Read the model definition and answer for the solid it produces. Units are mm, in the model's axes. Give positions to 0.01 mm unless a question says otherwise; leave off trailing zeros. Order: outer loops, then holes, each group sorted by start corner. A loop starts at its lowest first (then second) coordinate and runs counter-clockwise, first axis right, second up. Notation, with made-up numbers: M 74.25,75 L 121.25,75 A32 cw 121.25,107 Z; hole C 58.5,-7 d4. An arc over 180 degrees is marked long. Write item = value, one per line. Start each with the question number.
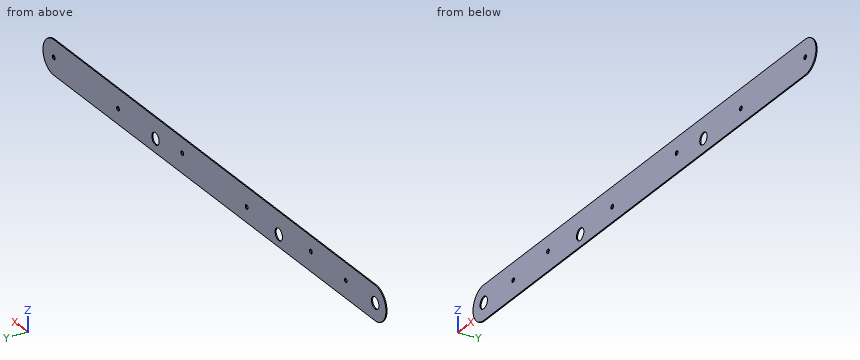
from build123d import *

# Parameters (mm, degrees)
F0_R     = 17.4625
F0_R_2   = 6.35
F1_DEPTH = 3.175


# Not quite as in the source:
# - a feature names something its author has since deleted; it is built from what else it names


with BuildPart() as f1:
    # F0 (on Front) → F1 (new body)
    with BuildSketch(Plane.XZ):
        with BuildLine():
            Line((0, -101.6), (1524, -101.6))
            Line((1524, -101.6), (1524, -57.15))
            ThreePointArc((1524, -57.15), (1517.65, -50.8), (1524, -44.45))
            Line((1524, -44.45), (1524, 0))
            Line((1524, 0), (0, 0))
            ThreePointArc((0, 0), (-35.9210244843, -14.8789755157), (-50.8, -50.8))
            ThreePointArc((-50.8, -50.8), (-35.9210244843, -86.7210244843), (0, -101.6))
        make_face()
        with BuildLine():
            ThreePointArc((17.4625, -50.8), (0, -68.2625), (-17.4625, -50.8))
            ThreePointArc((-17.4625, -50.8), (0, -33.3375), (17.4625, -50.8))
        make_face(mode=Mode.SUBTRACT)
        with BuildLine():
            ThreePointArc((145.7015722418, -50.8), (139.7015722418, -56.8), (133.7015722418, -50.8))
            ThreePointArc((133.7015722418, -50.8), (139.7015722418, -44.8), (145.7015722418, -50.8))
        make_face(mode=Mode.SUBTRACT)
        with Locations((457.2, -65.8510252833)):
            Circle(F0_R, mode=Mode.SUBTRACT)
        with Locations((609.6, -57.15)):
            Circle(F0_R_2, mode=Mode.SUBTRACT)
        with Locations((1041.4, -61.3564662635)):
            Circle(F0_R, mode=Mode.SUBTRACT)
        with Locations((1219.2, -57.15)):
            Circle(F0_R_2, mode=Mode.SUBTRACT)
        with Locations((304.8, -44.45)):
            Circle(F0_R_2, mode=Mode.SUBTRACT)
        with Locations((914.4, -44.45)):
            Circle(F0_R_2, mode=Mode.SUBTRACT)
        with BuildLine():
            Line((1524, -57.15), (1524, -101.6))
            ThreePointArc((1524, -101.6), (1574.8, -50.8), (1524, 0))
            Line((1524, 0), (1524, -44.45))
            ThreePointArc((1524, -44.45), (1528.4901280605, -46.3098719395), (1530.35, -50.8))
            ThreePointArc((1530.35, -50.8), (1528.4901280605, -55.2901280605), (1524, -57.15))
        make_face()
    extrude(amount=F1_DEPTH)


solid = f1.part
1) This flat-tipped pin is pushed along its axis until it touches: P1, Ø1, axis at y = -0.5, z = -82, coming from the -X side. Where does it stop, or does it pass through?
2) Find section A-A on x = 1041.4. Determine the outline of the cut face in (y, z) (3 decimals).
3) Find the intervals of material crossed by probe 1 along Z at (x, y) = (609.6, -1.95); probe 2 along Z at (x, y) = (1041.4, -2.5); probe 3 along X at (y, z) = (-2.15, -63), in increasing order. Write a range as [from, to].
4) Find section B-B on y = -0.6. Count the separate pieces of the cut face and the enclosed holes in it, plus the area to 3 significant figures.
Numbers:
q1.P1 = -40.47
q2.outline = M -3.175,-101.6 L 0,-101.6 L 0,-78.819 L -3.175,-78.819 Z; M -3.175,-43.894 L 0,-43.894 L 0,0 L -3.175,0 Z
q3.probe_1 = [-101.6, -63.5], [-50.8, 0]
q3.probe_2 = [-101.6, -78.82], [-43.89, 0]
q3.probe_3 = [-49.31, -12.49], [12.49, 439.97], [474.43, 607.13], [612.07, 1024.02], [1058.78, 1216.73], [1221.67, 1573.31]
q4.separate_pieces = 1
q4.enclosed_holes = 9
q4.area = 159,000 mm2
